Build history of the part. All positions in model axes, mm. A direction names the side the tool comes from. Round coordinates to 2 decimals unless told otherwise and drop trailing zeros. Order: outer loops, then holes, each group sorted by start corner. A loop starts at its lowest first (then second) coordinate and runs counter-clockwise, first axis right, second up. Notation, with made-up numbers: (-19, 48) -> (33, 48) arc R28 ccw to (33, 87) -> close; hole circle Ø2 at (60.25, -8). An arc over 180 degrees is marked (long way). Use a Markdown table: item, result. Add a question column.
Item 1: Slice it at C-C, the plane y = 3.2. State how many separate pieces and enclosed holes the cut face has, plus the area to 3 significant figures.
Item 2: Slice it at D-D, the plane x = -33. Give the cut face in (y, z).
Item 3: Pin check, flat tips, straight feed: pin 1 (3.5 mm diameter, centred on x = 13.96, z = 10.95, fed in from +Y); pin 2 (3 mm diameter, centred on x = 3, y = 4.5, fed in from -Z). Stop position of each tip, or through.
Item 4: Two-plate mould, pull along Z, no slides. Class faces 3 (the face through (15.57, 2.46, 25.99)), 4 (the face through (-0.725, 2.465, 25.254)): released by +Z, released by -Z, zero draft, split by the parting line, or undercut.
Item 5: 3-axis set-ups, long thin cutter, end or side, ignore diameter. For faces 1 (the face through (-29.559, 2.465, 24.748)), 2 (the face through (-22.91, 2.46, -26.07)): which of +Z, -Z, +X, -X, +Y, -Y reach the whole face in a straight line?
Item 6: Slice it at B-B, the plane z = -37. Give the cut face in (x, y).
Item 7: Probe L1, parallel to X at y = 0.5, z = -22; L2, parallel to Z at x = -27, y = 4.2; L3, parallel to X at y = 0.3, z = -24. List the from-to ranges inside material, lowest first.
Item 8: Slice it at A-A, the plane x = 21. Give the cut face in (y, z).
from build123d import *

# Parameters (mm, degrees)
SKETCH2_R           = 10
SKETCH2_R_2         = 2
BOSS_EXTRUDE1_DEPTH = 5


with BuildPart() as part:
    # Sketch2 → Boss-Extrude1 (new body)
    with BuildSketch(Plane(origin=(0, 0, 0), x_dir=(1, 0, 0), z_dir=(0, 1, 0))):
        with BuildLine():
            Line((18.784202094, 41.553321118), (36.461871623, 23.875651588))
            ThreePointArc((36.461871623, 23.875651588), (28.251193505, 4.053321118), (36.461871623, -15.769009352))
            Line((36.461871623, -15.769009352), (18.784202094, -33.446678882))
            ThreePointArc((18.784202094, -33.446678882), (-1.033353761, -25.252275183), (-20.844173422, -33.462950938))
            Line((-20.844173422, -33.462950938), (-38.521842951, -15.785281409))
            ThreePointArc((-38.521842951, -15.785281409), (-30.311167196, 4.048559871), (-38.538128377, 23.875651588))
            Line((-38.538128377, 23.875651588), (-20.860458847, 41.553321118))
            ThreePointArc((-20.860458847, 41.553321118), (-1.038128377, 33.342642999), (18.784202094, 41.553321118))
        make_face()
        with Locations(Location((-1.038128377, 4.053321118, 0), (0, 0, 270))):
            Circle(SKETCH2_R, mode=Mode.SUBTRACT)
        with Locations(Location((-16.038128377, 19.053321118, 0), (0, 0, 270))):
            Circle(SKETCH2_R_2, mode=Mode.SUBTRACT)
        with Locations(Location((13.961871623, 19.053321118, 0), (0, 0, 270))):
            Circle(SKETCH2_R_2, mode=Mode.SUBTRACT)
        with Locations(Location((13.961871623, -10.946678882, 0), (0, 0, 270))):
            Circle(SKETCH2_R_2, mode=Mode.SUBTRACT)
        with Locations(Location((-16.038128377, -10.946678882, 0), (0, 0, 270))):
            Circle(SKETCH2_R_2, mode=Mode.SUBTRACT)
        with BuildLine():
            Line((-17.678478332, 31.300272791), (-28.28508005, 20.693671073))
            ThreePointArc((-28.28508005, 20.693671073), (-31.113507174, 20.693671073), (-31.113507174, 23.522098198))
            Line((-31.113507174, 23.522098198), (-20.506905456, 34.128699916))
            ThreePointArc((-20.506905456, 34.128699916), (-17.678478332, 34.128699916), (-17.678478332, 31.300272791))
        make_face(mode=Mode.SUBTRACT)
        with BuildLine():
            Line((29.037250421, 23.522098198), (18.430648703, 34.128699916))
            ThreePointArc((18.430648703, 34.128699916), (15.602221578, 34.128699916), (15.602221578, 31.300272791))
            Line((15.602221578, 31.300272791), (26.208823296, 20.693671073))
            ThreePointArc((26.208823296, 20.693671073), (29.037250421, 20.693671073), (29.037250421, 23.522098198))
        make_face(mode=Mode.SUBTRACT)
        with BuildLine():
            Line((18.430648703, -26.022057679), (29.037250421, -15.415455962))
            ThreePointArc((29.037250421, -15.415455962), (29.037250421, -12.587028837), (26.208823296, -12.587028837))
            Line((26.208823296, -12.587028837), (15.602221578, -23.193630555))
            ThreePointArc((15.602221578, -23.193630555), (15.602221578, -26.022057679), (18.430648703, -26.022057679))
        make_face(mode=Mode.SUBTRACT)
        with BuildLine():
            Line((-31.113507174, -15.415455962), (-20.506905456, -26.022057679))
            ThreePointArc((-20.506905456, -26.022057679), (-17.678478332, -26.022057679), (-17.678478332, -23.193630555))
            Line((-17.678478332, -23.193630555), (-28.28508005, -12.587028837))
            ThreePointArc((-28.28508005, -12.587028837), (-31.113507174, -12.587028837), (-31.113507174, -15.415455962))
        make_face(mode=Mode.SUBTRACT)
    extrude(amount=BOSS_EXTRUDE1_DEPTH)


solid = part.part
Check sheet entries:
| question | item | result |
|---|---|---|
| 1 | separate pieces | 1 |
| 1 | enclosed holes | 9 |
| 1 | area | 3,450 mm2 |
| 2 | outline | (0, -29.41) -> (5, -29.41) -> (5, -16.02) -> (0, -16.02) -> close; (0, 7.94) -> (5, 7.94) -> (5, 21.31) -> (0, 21.31) -> close |
| 3 | pin 1 | through |
| 3 | pin 2 | z = -33.9 |
| 4 | face 3 | undercut |
| 4 | face 4 | released by +Z |
| 5 | face 1 | +Z, -X, +Y, -Y |
| 5 | face 2 | +Y, -Y |
| 6 | outline | (-25.41, 0) -> (-14.88, 0) -> (-14.88, 5) -> (-25.41, 5) -> close; (12.81, 0) -> (23.34, 0) -> (23.34, 5) -> (12.81, 5) -> close |
| 7 | L1 | -36.82 to -31.7, -26.98 to 24.9, 29.62 to 34.75 |
| 7 | L2 | -35.41 to -27.64, -21.98 to 13.87, 19.53 to 27.31 |
| 7 | L3 | -38.41 to -30.64, -24.98 to 22.9, 28.56 to 36.34 |
| 8 | outline | (0, -39.34) -> (5, -39.34) -> (5, -31.56) -> (0, -31.56) -> close; (0, -25.9) -> (5, -25.9) -> (5, 17.8) -> (0, 17.8) -> close; (0, 23.45) -> (5, 23.45) -> (5, 31.23) -> (0, 31.23) -> close |
